from build123d import *

# Parameters (mm, degrees)
F0_W     = 6.35
F0_H     = 6.35
F1_DEPTH = 6.35


with BuildPart() as f1:
    # F0 (on Top) → F1 (new body)
    with BuildSketch(Plane.XY):
        Polygon((76.2, 50.8), (76.2, 63.5), (69.85, 63.5), (69.85, 57.15), (63.5, 57.15), (57.15, 57.15), (50.8, 57.15), (44.45, 57.15), (44.45, 63.5), (38.1, 63.5), (31.75, 63.5), (25.4, 63.5), (19.05, 63.5), (19.05, 57.15), (-19.05, 57.15), (-19.05, 63.5), (-25.4, 63.5), (-31.75, 63.5), (-38.1, 63.5), (-44.45, 63.5), (-44.45, 57.15), (-69.85, 57.15), (-69.85, 63.5), (-76.2, 63.5), (-76.2, 50.8), (-76.2, 44.45), (-69.85, 44.45), (-69.85, 38.1), (-76.2, 38.1), (-76.2, 31.75), (-69.85, 31.75), (-69.85, 25.4), (-76.2, 25.4), (-76.2, 19.05), (-69.85, 19.05), (-69.85, 12.7), (-76.2, 12.7), (-76.2, 6.35), (-69.85, 6.35), (-69.85, 0), (-76.2, 0), (-76.2, -6.35), (-69.85, -6.35), (-69.85, -12.7), (-76.2, -12.7), (-76.2, -19.05), (-69.85, -19.05), (-69.85, -25.4), (-76.2, -25.4), (-76.2, -31.75), (-69.85, -31.75), (-69.85, -38.1), (-76.2, -38.1), (-76.2, -44.45), (-69.85, -44.45), (-69.85, -50.8), (-76.2, -50.8), (-76.2, -57.15), (-69.85, -57.15), (-50.8, -57.15), (-50.8, -63.5), (-44.45, -63.5), (-38.1, -63.5), (-31.75, -63.5), (-25.4, -63.5), (-25.4, -57.15), (-19.05, -57.15), (-12.7, -57.15), (-6.35, -57.15), (0, -57.15), (6.35, -57.15), (12.7, -57.15), (19.05, -57.15), (25.4, -57.15), (25.4, -63.5), (31.75, -63.5), (38.1, -63.5), (44.45, -63.5), (50.8, -63.5), (50.8, -57.15), (57.15, -57.15), (69.85, -57.15), (69.85, -63.5), (76.2, -63.5), (76.2, -50.8), (76.2, -44.45), (76.2, -38.1), (76.2, -31.75), (76.2, -25.4), (-63.5, -25.4), (-63.5, 25.4), (76.2, 25.4), (76.2, 31.75), (76.2, 38.1), (76.2, 44.45), align=None)
        with Locations((-73.025, 41.275)):
            Rectangle(F0_W, F0_H)
        with Locations((-73.025, 28.575)):
            Rectangle(F0_W, F0_H)
        with Locations((-73.025, 15.875)):
            Rectangle(F0_W, F0_H)
        with Locations((-73.025, 3.175)):
            Rectangle(F0_W, F0_H)
        with Locations((-73.025, -9.525)):
            Rectangle(F0_W, F0_H)
        with Locations((-73.025, -22.225)):
            Rectangle(F0_W, F0_H)
        with Locations((-73.025, -34.925)):
            Rectangle(F0_W, F0_H)
        with Locations((-73.025, -47.625)):
            Rectangle(F0_W, F0_H)
    extrude(amount=F1_DEPTH)


solid = f1.part
Read the model definition and answer for the solid it produces. Units are mm, in the model's axes. A direction names the side the tool comes from. Coordinates: 2 decimals unless noted, no trailing zeros. Loops run counter-clockwise (first coordinate to the right, second up) from the corner with the lowest first, then second, coordinate; pieces in that order, holes last. Notation, with made-up numbers: (53, 2.5) -> (59, 2.5) arc R21 cw to (59, 37.5) -> close; hole circle Ø2 at (-12, 80). An arc over 180 degrees is marked (long way). Write item = value, one per line. Start each with the question number.
1) The part is cut by section A-A, the plane x = -28.5. Determine the outline of the cut face in (y, z).
2) The mould has two halves that part along Y. Classify faces 1 (the face through (5, 25.4, 3)), 2 (the face through (-19.05, 60, 3)), 3 (the face through (73, 63.5, 3)): pulls with the +Y half, pulls with the -Y half, needs draft (parallel to the pull), parting line crosses it, or undercut.
3) Given P1, Ø1.9, axis at y = -8, z = 2, coming from the +X side; P2, Ø3, axis at y = -59, z = 4, coming from the -X side; P3, Ø1.9, axis at x = -55, z = 3.5, coming from the +Y side, each flat-ended and moving along its own axis, determine where each tip first touches the part or whether it passes through.
4) Find the intervals of material crossed by L1, parallel to Y at x = -51, z = 6.25; L2, parallel to Y at x = -23.5, z = 5.25; L3, parallel to X at y = -23.5, z = 0.75, in increasing order. Write a range as from..to.
5) The part is cut by section C-C, the plane y = 2. Determine the outline of the cut face in (x, z), plus the area to 3 significant figures.
6) For faces 4 (the face through (-57, 57.15, 3)), 5 (the face through (-64, -57.15, 3)), 6 (the face through (-63.5, 0, 3)), 7 (the face through (60, -57.15, 3)), determine the directions among +Z, -Z, +X, -X, +Y, -Y from which every point of the face is accessible in a straight line to the end or side of a thin tool.
Result:
q1.outline = (-63.5, 0) -> (-25.4, 0) -> (-25.4, 6.35) -> (-63.5, 6.35) -> close; (25.4, 0) -> (63.5, 0) -> (63.5, 6.35) -> (25.4, 6.35) -> close
q2.face_1 = undercut
q2.face_2 = needs draft
q2.face_3 = pulls with the +Y half
q3.P1 = -63.5
q3.P2 = -50.8
q3.P3 = 57.15
q4.L1 = -57.15..-25.4, 25.4..57.15
q4.L2 = -57.15..-25.4, 25.4..63.5
q4.L3 = -76.2..-63.5
q5.outline = (-76.2, 0) -> (-63.5, 0) -> (-63.5, 6.35) -> (-76.2, 6.35) -> close
q5.area = 80.6 mm²
q6.face_4 = +Z, -Z, +Y
q6.face_5 = +Z, -Z, -X, -Y
q6.face_6 = +Z, -Z, +X
q6.face_7 = +Z, -Z, -Y
